```python
from build123d import *

# Parameters (mm, degrees)
SKETCH_1_R      = 12.5
SKETCH_1_R_2    = 5
EXTRUDE_1_DEPTH = 80
FILLET_1_R      = 3
FILLET_2_R      = 2
FILLET_3_R      = 2


with BuildPart() as part:
    # Эскиз1 → Вытянуть-Тонкостенный1 (new body)
    with BuildSketch(Plane.XY):
        Circle(SKETCH_1_R)
        Circle(SKETCH_1_R_2, mode=Mode.SUBTRACT)
    extrude(amount=EXTRUDE_1_DEPTH)

    # Эскиз2 → Вырез-Повернуть1 (revolve, cut)
    with BuildSketch(Plane(origin=(0, 0, 0), x_dir=(1, 0, 0), z_dir=(0, 1, 0)), mode=Mode.PRIVATE) as cut_revolve_1_sk:
        Polygon((12.5, -10), (8.5, -10), (12.5, -25), align=None)
    revolve(cut_revolve_1_sk.sketch.rotate(Axis((0, 0, -6.599641281), (0, 0, 1)), 180), axis=Axis((0, 0, -6.599641281), (0, 0, 1)), mode=Mode.SUBTRACT)

    # Скругление1
    fillet_1_edges = [part.edges().sort_by_distance(p)[0] for p in [
        (-12.5, 0, 10),
    ]]
    fillet(fillet_1_edges, radius=FILLET_1_R)

    # Скругление2
    fillet_2_edges = [part.edges().sort_by_distance(p)[0] for p in [
        (8.5, 0, 10),
    ]]
    fillet(fillet_2_edges, radius=FILLET_2_R)

    # Скругление3
    fillet_3_edges = [part.edges().sort_by_distance(p)[0] for p in [
        (0, -12.5, 25),
    ]]
    fillet(fillet_3_edges, radius=FILLET_3_R)


solid = part.part
```
Input: part model. Units: mm. Frame: model coordinates. Coordinates: 2 decimals unless noted, no trailing zeros. Loops run counter-clockwise (first coordinate to the right, second up) from the corner with the lowest first, then second, coordinate; pieces in that order, holes last. Notation, with made-up numbers: M 60.25,-17.75 L 87.25,-17.75 A19 ccw 87.25,14.25 Z; hole C -35,67 d3. An arc over 180 degrees is marked long. Answer in a Markdown table with one row per item.
1. Draft query along Z for faces 1 (the flat face through (-0.2, -5.4, 80)), 2 (the flat face through (-0.2, -5.4, 0)), 3 (the conical face through (-9.59, -3.02, 15.83)), 4 (the cylindrical face through (-1.08, -4.88, 39.44)). Return one class per face: pulls with the +Z half, pulls with the -Z half, needs draft (parallel to the pull), parting line crosses it, or undercut.
Response:
| item | result |
|---|---|
| face 1 | pulls with the +Z half |
| face 2 | pulls with the -Z half |
| face 3 | undercut |
| face 4 | needs draft |
2. Section A-A, the plane z = 73.5. Output: boundary loops of the cut face in (x, y).
Response:
| item | result |
|---|---|
| outline | C 0,0 d25; hole C 0,0 d10 |
3. First-contact query: pin 1 (10 mm diameter, centred on x = 8, z = 13, fed in from +Y); pin 2 (8 mm diameter, centred on y = 4.5, z = 65, fed in from -X); pin 3 (1 mm diameter, centred on x = -8.5, z = 28, fed in from -Y); pin 4 (8 mm diameter, centred on x = 2.5, z = 29, fed in from +Y). Flat tips, straight axial feed; report the tip coordinate or a pass-through.
Response:
| item | result |
|---|---|
| pin 1 | stops at y = 10.66 |
| pin 2 | stops at x = -12.49 |
| pin 3 | stops at y = -9.6 |
| pin 4 | stops at y = 12.5 |
4. Section B-B, the plane z = 19. Output: boundary loops of the cut face in (x, y), then the cut area to 3 significant figures.
Response:
| item | result |
|---|---|
| outline | C 0,0 d21.8; hole C 0,0 d10 |
| area | 295 mm2 |
5. Material intervals for line 1 (Y direction, x = 0, z = 50.5); line 2 (X direction, y = -3.5, z = 51.5); line 3 (Y direction, x = -2.25, z = 49), sorted ascending.
Response:
| item | result |
|---|---|
| line 1 | y = -12.5 to -5, 5 to 12.5 |
| line 2 | x = -12 to -3.57, 3.57 to 12 |
| line 3 | y = -12.3 to -4.47, 4.47 to 12.3 |
